Here's the drawing with two shaded views (mm, measured from the low corner). I have some questions. Round coordinates to 2 decimals unless told otherwise and drop trailing zeros. Order: outer loops, then holes, each group sorted by start corner. A loop starts at its lowest first (then second) coordinate and runs counter-clockwise, first axis right, second up.
Q1. If we section it at D-D (y = 7.4): Please give me the cut outline in (x, z), plus the area to 3 significant figures.
Q2. We'd pull the mould along Y, two halves only. Please class the marked faces 1 and 2: pulls with the +Y half, pulls with the -Y half, needs draft (parallel to the pull), parting line crosses it, or undercut.
Q3. If we section it at B-B (x = 17.5): Please give me the cut outline in (y, z).
Q4. If we section it at C-C (z = 1.75): Please give me the cut outline in (x, y), plus the area to 3 significant figures.
Q5. If I drill on line 1 (X direction, y = 5.5, z = 0.75); line 2 (Y direction, x = 17.5, z = 1.7); line 3 (X direction, y = 8, z = 0.35), over which ranges is the centre line in solid material (lowest first)?
Q6. If we section it at A-A (y = 4.35): Please give me the cut outline in (x, z), plus the area to 3 significant figures.
Q7. Will this pin go through, and if not, where does the flat tip stop? P1, Ø0.6, axis at x = 3, z = 1, coming from the +Y side.
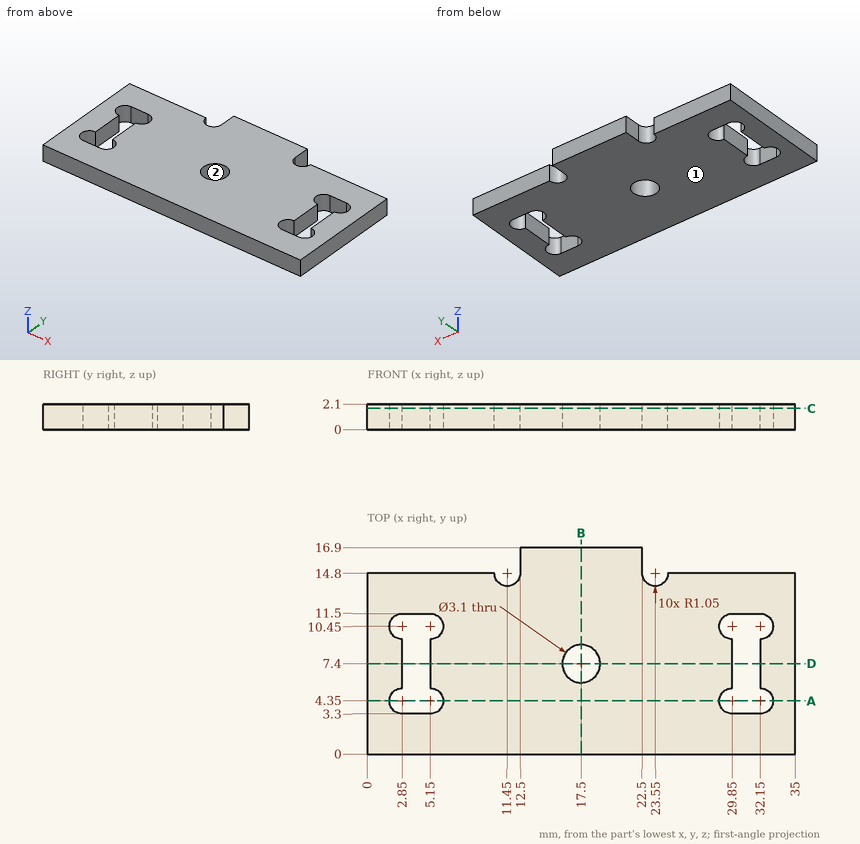
Solution:
1. outline: (0, 0) - (2.85, 0) - (2.85, 2.1) - (0, 2.1) - close; (5.15, 0) - (15.95, 0) - (15.95, 2.1) - (5.15, 2.1) - close; (19.05, 0) - (29.85, 0) - (29.85, 2.1) - (19.05, 2.1) - close; (32.15, 0) - (35, 0) - (35, 2.1) - (32.15, 2.1) - close
1. area: 57.3 mm2
2. face 1: needs draft
2. face 2: undercut
3. outline: (0, 0) - (5.85, 0) - (5.85, 2.1) - (0, 2.1) - close; (8.95, 0) - (16.9, 0) - (16.9, 2.1) - (8.95, 2.1) - close
4. outline: (0, 0) - (35, 0) - (35, 14.8) - (24.6, 14.8) arc R1.05 cw to (22.5, 14.8) - (22.5, 16.9) - (12.5, 16.9) - (12.5, 14.8) arc R1.05 cw to (10.4, 14.8) - (0, 14.8) - close; hole (2.85, 3.3) - (5.15, 3.3) arc R1.05 ccw to (5.15, 5.4) - (5.15, 9.4) arc R1.05 ccw to (5.15, 11.5) - (2.85, 11.5) arc R1.05 ccw to (2.85, 9.4) - (2.85, 5.4) arc R1.05 ccw to start; hole circle Ø3.1 at (17.5, 7.4); hole (29.85, 3.3) - (32.15, 3.3) arc R1.05 ccw to (32.15, 5.4) - (32.15, 9.4) arc R1.05 ccw to (32.15, 11.5) - (29.85, 11.5) arc R1.05 ccw to (29.85, 9.4) - (29.85, 5.4) arc R1.05 ccw to start
4. area: 476 mm2
5. line 1: x = 0 to 2.85, 5.15 to 29.85, 32.15 to 35
5. line 2: y = 0 to 5.85, 8.95 to 16.9
5. line 3: x = 0 to 2.85, 5.15 to 16.07, 18.93 to 29.85, 32.15 to 35
6. outline: (0, 0) - (1.8, 0) - (1.8, 2.1) - (0, 2.1) - close; (6.2, 0) - (28.8, 0) - (28.8, 2.1) - (6.2, 2.1) - close; (33.2, 0) - (35, 0) - (35, 2.1) - (33.2, 2.1) - close
6. area: 55.0 mm2
7. P1: stops at y = 14.8
